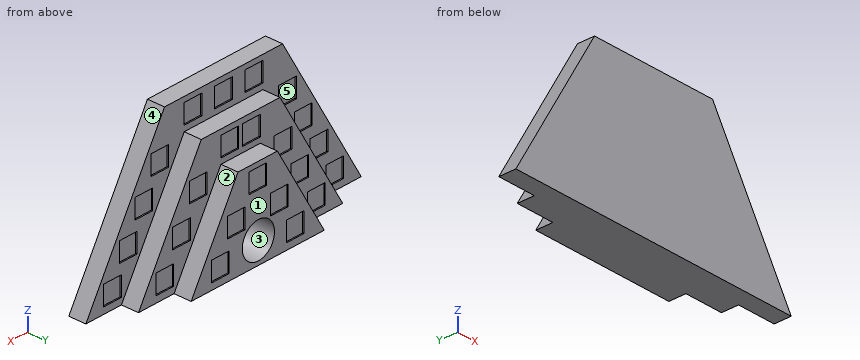
```python
from build123d import *

# Parameters (mm, degrees)
BOSS_EXTRUDE1_DEPTH = 40
BOSS_EXTRUDE2_DEPTH = 40
BOSS_EXTRUDE3_DEPTH = 80
SKETCH7_W           = 45
SKETCH7_H           = 45
CUT_EXTRUDE2_DEPTH  = 3
SKETCH8_W           = 45
SKETCH8_H           = 45
CUT_EXTRUDE3_DEPTH  = 3
SKETCH9_W           = 45
SKETCH9_H           = 45
CUT_EXTRUDE4_DEPTH  = 3
SKETCH11_W          = 45
SKETCH11_H          = 45
CUT_EXTRUDE5_DEPTH  = 3
SKETCH13_R          = 41
CUT_EXTRUDE6_DEPTH  = 117


with BuildPart() as part:
    # Sketch1 → Boss-Extrude1 (new body)
    with BuildSketch(Plane(origin=(0, 0, 0), x_dir=(1, 0, 0), z_dir=(0, 1, 0))):
        Polygon((-150, 0), (150, 0), (350, 346.410161514), (-350, 346.410161514), align=None)
    extrude(amount=BOSS_EXTRUDE1_DEPTH)

    # Sketch3 → Boss-Extrude2 (add)
    with BuildSketch(Plane(origin=(0, 40, 0), x_dir=(1, 0, 0), z_dir=(0, 1, 0))):
        Polygon((-100, 70), (100, 70), (259.585481157, 346.410161514), (169.170962313, 346.410161514), (50, 140), (-50, 140), (-169.170962313, 346.410161514), (-259.585481157, 346.410161514), align=None)
    extrude(amount=BOSS_EXTRUDE2_DEPTH)

    # Sketch4 → Boss-Extrude3 (add)
    with BuildSketch(Plane(origin=(0, 40, 0), x_dir=(1, 0, 0), z_dir=(0, 1, 0))):
        Polygon((169.170962313, 346.410161514), (-169.170962313, 346.410161514), (-50, 140), (50, 140), align=None)
    extrude(amount=BOSS_EXTRUDE3_DEPTH)

    # Sketch7 → Cut-Extrude2 (cut)
    with BuildSketch(Plane(origin=(0, 40, 0), x_dir=(1, 0, 0), z_dir=(0, 1, 0))):
        with Locations((-282.5, 308.910161514)):
            Rectangle(SKETCH7_W, SKETCH7_H)
        with Locations((-77.5, 34.5)):
            Rectangle(SKETCH7_W, SKETCH7_H)
        with Locations((-242.5, 239.628129211)):
            Rectangle(SKETCH7_W, SKETCH7_H)
        with Locations((-202.5, 170.346096908)):
            Rectangle(SKETCH7_W, SKETCH7_H)
        with Locations((-162.5, 101.064064606)):
            Rectangle(SKETCH7_W, SKETCH7_H)
        with Locations((282.5, 308.910161514)):
            Rectangle(SKETCH7_W, SKETCH7_H)
        with Locations((162.5, 101.064064606)):
            Rectangle(SKETCH7_W, SKETCH7_H)
        with Locations((202.5, 170.346096908)):
            Rectangle(SKETCH7_W, SKETCH7_H)
        with Locations((242.5, 239.628129211)):
            Rectangle(SKETCH7_W, SKETCH7_H)
        with Locations((0, 34.5)):
            Rectangle(SKETCH7_W, SKETCH7_H)
        with Locations((77.5, 34.5)):
            Rectangle(SKETCH7_W, SKETCH7_H)
    extrude(amount=-CUT_EXTRUDE2_DEPTH, mode=Mode.SUBTRACT)

    # Sketch8 → Cut-Extrude3 (cut)
    with BuildSketch(Plane(origin=(0, 80, 0), x_dir=(1, 0, 0), z_dir=(0, 1, 0))):
        with Locations((-192.5, 308.910161514)):
            Rectangle(SKETCH8_W, SKETCH8_H)
        with Locations((-150.235026919, 235.705080757)):
            Rectangle(SKETCH8_W, SKETCH8_H)
        with Locations((-107.970053838, 162.5)):
            Rectangle(SKETCH8_W, SKETCH8_H)
        with Locations((192.5, 308.910161514)):
            Rectangle(SKETCH8_W, SKETCH8_H)
        with Locations((150.235026919, 235.705080757)):
            Rectangle(SKETCH8_W, SKETCH8_H)
        with Locations((107.970053838, 162.5)):
            Rectangle(SKETCH8_W, SKETCH8_H)
    extrude(amount=-CUT_EXTRUDE3_DEPTH, mode=Mode.SUBTRACT)

    # Sketch9 → Cut-Extrude4 (cut)
    with BuildSketch(Plane(origin=(0, 80, 0), x_dir=(1, 0, 0), z_dir=(0, 1, 0))):
        with Locations((-27.5, 105)):
            Rectangle(SKETCH9_W, SKETCH9_H)
        with Locations((27.5, 105)):
            Rectangle(SKETCH9_W, SKETCH9_H)
    extrude(amount=-CUT_EXTRUDE4_DEPTH, mode=Mode.SUBTRACT)

    # Sketch11 → Cut-Extrude5 (cut)
    with BuildSketch(Plane(origin=(0, 120, 0), x_dir=(1, 0, 0), z_dir=(0, 1, 0))):
        with Locations((-54.820508076, 238.910161514)):
            Rectangle(SKETCH11_W, SKETCH11_H)
        with Locations((-95.235026919, 308.910161514)):
            Rectangle(SKETCH11_W, SKETCH11_H)
        with Locations((54.820508076, 238.910161514)):
            Rectangle(SKETCH11_W, SKETCH11_H)
        with Locations((95.235026919, 308.910161514)):
            Rectangle(SKETCH11_W, SKETCH11_H)
        with Locations((0, 173.910161514)):
            Rectangle(SKETCH11_W, SKETCH11_H)
    extrude(amount=-CUT_EXTRUDE5_DEPTH, mode=Mode.SUBTRACT)

    # Sketch13 → Cut-Extrude6 (cut)
    with BuildSketch(Plane(origin=(0, 120, 0), x_dir=(1, 0, 0), z_dir=(0, 1, 0))):
        with Locations((-1.735026919, 296.410161514)):
            Circle(SKETCH13_R)
    extrude(amount=-CUT_EXTRUDE6_DEPTH, mode=Mode.SUBTRACT)


solid = part.part
```
Can you work these out from the model? Positions are in its coordinate system, mm. Face numbers are marked on the shaded views. A direction names the side the tool comes from. Coordinates: 2 decimals unless noted, no trailing zeros. Loops run counter-clockwise (first coordinate to the right, second up) from the corner with the lowest first, then second, coordinate; pieces in that order, holes last. Notation, with made-up numbers: M -4.5,63.25 L 20.5,63.25 A18 cw 20.5,83.25 Z; hole C -28,13 d6. An arc over 180 degrees is marked long. Put each result on its own line as item: value. Start each with the question number.
(1) We'd pull the mould along Z, two halves only. Please class the marked faces 1, 2 and 3: +Z half, -Z half, draft (parallel to the pull), parting line (faces both ways), or undercut.
(2) Will these pins go through, and if not, where does the flat tip stop? pin 1 Ø13.5 at (x, z) = (101.5, -309.5) entering from +Y; pin 2 Ø10 at (y, z) = (59, -225) entering from -X; pin 3 Ø1.5 at (x, y) = (274, 39) entering from +Z.
(3) Imagine slicing it at D-D on x = 63.5. List the corners of the cut face in (y, z) for me.
(4) Imagine slicing it at B-B on z = -114.5. List the corners of the cut face in (x, y) for me, and give its area (3 significant figures).
(5) Which directions (+Z, -Z, +X, -X, +Y, -Y) give clear straight access to the entire face, cutting with the end or side of a thin tool? Please do the marked faces 4 and 5.
(6) I need wall thicknesses on probe 1 along Y at (x, z) = (21, -165); probe 2 along Y at (x, z) = (-131, -18.5); probe 3 along X at (y, z) = (94.5, -325). Which ranges of each line are inside material? Lowest first, please.
(7) Imagine slicing it at A-A on x = 253. List the corners of the cut face in (y, z) for me, and give its area (3 significant figures).
(8) Imagine slicing it at C-C on y = 67.5. List the corners of the cut face in (x, z) for me, and give its area (3 significant figures).
Worked answers:
1. face 1: draft
1. face 2: +Z half
1. face 3: undercut
2. pin 1: stops at y = 117
2. pin 2: stops at x = -192.38
2. pin 3: stops at z = -213.48
3. outline: M 0,-346.41 L 120,-346.41 L 120,-261.41 L 117,-261.41 L 117,-216.41 L 120,-216.41 L 120,-163.38 L 80,-163.38 L 80,-70 L 40,-70 L 40,-57 L 37,-57 L 37,-12 L 40,-12 L 40,0 L 0,0 Z
4. outline: M -216.11,0 L 216.11,0 L 216.11,40 L 185,40 L 185,37 L 140,37 L 140,40 L 125.69,40 L 125.69,80 L 50,80 L 50,77 L 5,77 L 5,80 L -5,80 L -5,77 L -50,77 L -50,80 L -125.69,80 L -125.69,40 L -140,40 L -140,37 L -185,37 L -185,40 L -216.11,40 Z
4. area: 26,800 mm2
5. face 4: +Z, +X, +Y, -Y
5. face 5: +Y
6. probe 1: y = 0 to 117
6. probe 2: y = 0 to 40
6. probe 3: x = -156.81 to -31.12, 27.65 to 156.81
7. outline: M 0,-346.41 L 80,-346.41 L 80,-335 L 40,-335 L 40,-262.13 L 37,-262.13 L 37,-217.13 L 40,-217.13 L 40,-178.4 L 0,-178.4 Z
7. area: 7,040 mm2
8. outline: M -259.59,-346.41 L 259.59,-346.41 L 100,-70 L -100,-70 Z; hole C -1.74,-296.41 d82
8. area: 94,100 mm2
